Here's how the part is built. I have some questions about the finished solid (model axes, mm). Round coordinates to 2 decimals unless told otherwise and drop trailing zeros. Write each loop counter-clockwise with the first axis right and the second up, starting at its lowest first coordinate (ties: lowest second). Pieces come first, ordered by that corner, then holes. Notation, with made-up numbers: (6, 73) - (12, 73) arc R12 cw to (12, 95) - close; hole circle Ø1 at (-1, 48.25). An arc over 180 degrees is marked (long way). Return JSON: item names as keys, results as strings. Group by question number.
```python
from build123d import *

# Parameters (mm, degrees)
EXTRUDE_START   = 25
SKETCH_2_R      = 2
SKETCH_2_R_2    = 7.5
SKETCH_2_R_3    = 2.5
SKETCH_2_R_4    = 1.5
EXTRUDE_1_DEPTH = 2


with BuildPart() as part:
    # 草图2 → 凸台-拉伸1 (new body)
    with BuildSketch(Plane.XY.offset(EXTRUDE_START)):
        with BuildLine():
            Line((27, -3), (27, 2))
            Line((27, 2), (22.5, 2))
            Line((22.5, 2), (22.5, -3))
            Line((22.5, -3), (15, -3))
            ThreePointArc((15, -3), (6.514718626, -6.514718626), (3, -15))
            Line((3, -15), (3, -22.5))
            Line((3, -22.5), (-2, -22.5))
            Line((-2, -22.5), (-2, -27))
            Line((-2, -27), (15, -27))
            ThreePointArc((15, -27), (21, -25.392304845), (25.392304845, -21))
            Line((25.392304845, -21), (33, -21))
            Line((33, -21), (80.631397208, -48.5))
            Line((80.631397208, -48.5), (100.631397208, -48.5))
            Line((100.631397208, -48.5), (117.584077602, 26.706974803))
            Line((117.584077602, 26.706974803), (69.584077602, 26.842860701))
            Line((69.584077602, 26.842860701), (27, -3))
        make_face()
        with Locations((57, -15)):
            Circle(SKETCH_2_R, mode=Mode.SUBTRACT)
        with Locations((15, -15)):
            Circle(SKETCH_2_R_2, mode=Mode.SUBTRACT)
        with Locations((59, -28)):
            Circle(SKETCH_2_R_3, mode=Mode.SUBTRACT)
        with Locations((102.39866677, 8.999892909)):
            Circle(SKETCH_2_R_4, mode=Mode.SUBTRACT)
        with Locations((95.373546557, -21.983660567)):
            Circle(SKETCH_2_R_4, mode=Mode.SUBTRACT)
    extrude(amount=EXTRUDE_1_DEPTH)


solid = part.part
```
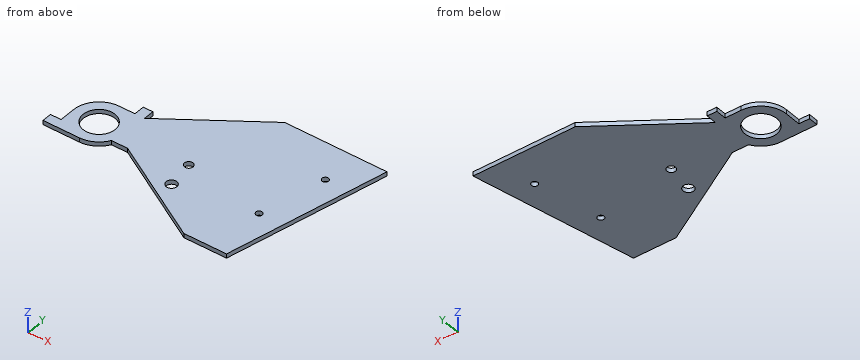
1) Imagine slicing it at A-A (y = -9.5). Please give me the cut outline in (x, z), plus the area to 3 significant figures.
2) Imagine slicing it at B-B (z = 25.8). Please give me the cut outline in (x, y).
3) Imagine slicing it at C-C (x = 106). Please give me the cut outline in (y, z), plus the area to 3 significant figures.
4) Will these pins go through, and if not, where does the flat tip stop? pin 1 Ø0.6 at (x, z) = (0.5, 26) entering from +Y; pin 2 Ø1 at (y, z) = (-34.5, 25) entering from +X; pin 3 Ø1 at (x, z) = (61, 26) entering from -Y.
5) I need wall thicknesses on line 1 along Y through (x, z) = (57.5, 26.7); line 2 along Y through (x, z) = (18, 25.35); line 3 along Y through (x, z) = (14, 25.85). Which ranges of each line are inside material? Lowest first, please.
Results found:
{
 "1": {"outline": "(4.33, 25) - (9.9, 25) - (9.9, 27) - (4.33, 27) - close; (20.1, 25) - (109.42, 25) - (109.42, 27) - (20.1, 27) - close", "area": "190 mm²"},
 "2": {"outline": "(-2, -27) - (15, -27) arc R12 ccw to (25.39, -21) - (33, -21) - (80.63, -48.5) - (100.63, -48.5) - (117.58, 26.71) - (69.58, 26.84) - (27, -3) - (27, 2) - (22.5, 2) - (22.5, -3) - (15, -3) arc R12 ccw to (3, -15) - (3, -22.5) - (-2, -22.5) - close; hole circle Ø15 at (15, -15); hole circle Ø4 at (57, -15); hole circle Ø5 at (59, -28); hole circle Ø3 at (95.37, -21.98); hole circle Ø3 at (102.4, 9)"},
 "3": {"outline": "(-24.68, 25) - (26.74, 25) - (26.74, 27) - (-24.68, 27) - close", "area": "103 mm²"},
 "4": {"pin 1": "stops at y = -22.5", "pin 2": "stops at x = 103.9", "pin 3": "stops at y = -37.45"},
 "5": {"line 1": "y = -35.15 to -30, -26 to -16.94, -13.06 to 18.37", "line 2": "y = -26.62 to -21.87, -8.13 to -3", "line 3": "y = -27 to -22.43, -7.57 to -3.04"}
}
